Verification items for the finished model (mm, model axes). A direction names the side the tool comes from. Give positions to 0.01 mm unless a question says otherwise; leave off trailing zeros. Loops run counter-clockwise (first coordinate to the right, second up) from the corner with the lowest first, then second, coordinate; pieces in that order, holes last. Notation, with made-up numbers: (32, 50) - (79, 50) arc R23 ccw to (79, 71) - close; hole circle Ø9 at (-15.5, -2). An arc over 180 degrees is marked (long way). Use one line per item in the form item = value.
```python
from build123d import *

# Parameters (mm, degrees)
AUFSATZ_LINEAR_AUSTRAGEN1_DEPTH                      = 10
SCHNITT_LINEAR_AUSTRAGEN1_DEPTH                      = 8
SCHNITT_LINEAR_AUSTRAGEN2_DEPTH                      = 6
SKIZZE4_W                                            = 12
SKIZZE4_H                                            = 12
AUFSATZ_LINEAR_AUSTRAGEN2_DEPTH                      = 5
FASE1_SIZE                                           = 5
FORMSENKUNG_F_R_M4_LINSENSENKSCHRAUBE_MI_D           = 4.5
FORMSENKUNG_F_R_M4_LINSENSENKSCHRAUBE_MI_CSINK_D     = 9.4
FORMSENKUNG_F_R_M4_LINSENSENKSCHRAUBE_MI_CSINK_ANGLE = 90
VERRUNDUNG1_R                                        = 2
SKIZZE8_W                                            = 10.4
SKIZZE8_H                                            = 2
AUFSATZ_LINEAR_AUSTRAGEN3_DEPTH                      = 1
FASE2_SIZE                                           = 2


with BuildPart() as part:
    # Skizze1 → Aufsatz-Linear austragen1 (new body)
    with BuildSketch(Plane.XY):
        Polygon((-12, 0), (12, 0), (12, -12), (24, -12), (24, -24), (-24, -24), (-24, -12), (-12, -12), align=None)
    extrude(amount=AUFSATZ_LINEAR_AUSTRAGEN1_DEPTH)

    # Skizze2 → Schnitt-Linear austragen1 (cut)
    with BuildSketch(Plane.XY.offset(10)):
        Polygon((-5.2, -1), (-5.2, -7), (-24, -7), (-24, -24), (24, -24), (24, -7), (5.2, -7), (5.2, -1), align=None)
    extrude(amount=-SCHNITT_LINEAR_AUSTRAGEN1_DEPTH, mode=Mode.SUBTRACT)

    # Skizze3 → Schnitt-Linear austragen2 (cut)
    with BuildSketch(Plane(origin=(0, 0, 0), x_dir=(1, 0, 0), z_dir=(0, 1, 0))):
        with BuildLine():
            Line((-2.75, -2.8), (2.75, -2.8))
            ThreePointArc((2.75, -2.8), (4.5, -4.55), (2.75, -6.3))
            Line((2.75, -6.3), (-2.75, -6.3))
            ThreePointArc((-2.75, -6.3), (-4.5, -4.55), (-2.75, -2.8))
        make_face()
    extrude(amount=-SCHNITT_LINEAR_AUSTRAGEN2_DEPTH, mode=Mode.SUBTRACT)

    # Skizze4 → Aufsatz-Linear austragen2 (add)
    with BuildSketch(Plane.XY.offset(2)):
        with Locations((-18, -18)):
            Rectangle(SKIZZE4_W, SKIZZE4_H)
        with Locations((18, -18)):
            Rectangle(SKIZZE4_W, SKIZZE4_H)
    extrude(amount=AUFSATZ_LINEAR_AUSTRAGEN2_DEPTH)

    # Fase1
    fase1_edges = [part.edges().sort_by_distance(p)[0] for p in [
        (12, -18, 2),
        (-12, -18, 2),
    ]]
    chamfer(fase1_edges, length=FASE1_SIZE - 0.0001)  # a hair under: the kernel refuses the full size

    # Formsenkung für M4 Linsensenkschraube mit Schlitz1 (through all)
    with Locations(Plane.XY.offset(7)):
        with Locations((-18, -18), (18, -18)):
            CounterSinkHole(FORMSENKUNG_F_R_M4_LINSENSENKSCHRAUBE_MI_D / 2, FORMSENKUNG_F_R_M4_LINSENSENKSCHRAUBE_MI_CSINK_D / 2, counter_sink_angle=FORMSENKUNG_F_R_M4_LINSENSENKSCHRAUBE_MI_CSINK_ANGLE)

    # Verrundung1
    verrundung1_edges = [part.edges().sort_by_distance(p)[0] for p in [
        (24, -12, 3.5),
        (24, -24, 3.5),
        (-24, -24, 3.5),
        (-24, -12, 3.5),
    ]]
    fillet(verrundung1_edges, radius=VERRUNDUNG1_R)

    # Skizze8 → Aufsatz-Linear austragen3 (add)
    with BuildSketch(Plane.XY.offset(10)):
        with Locations((0, -2)):
            Rectangle(SKIZZE8_W, SKIZZE8_H)
    extrude(amount=-AUFSATZ_LINEAR_AUSTRAGEN3_DEPTH)

    # Fase2
    fase2_edges = [part.edges().sort_by_distance(p)[0] for p in [
        (0, -1, 9),
    ]]
    chamfer(fase2_edges, length=FASE2_SIZE - 0.0001)  # a hair under: the kernel refuses the full size


solid = part.part
```
1. Section check C-C, the plane z = 1.25. Record the cut outline in (x, y).
Result set:
outline = (-24, -22) arc R2 ccw to (-22, -24) - (22, -24) arc R2 ccw to (24, -22) - (24, -14) arc R2 ccw to (22, -12) - (12, -12) - (12, 0) - (-12, 0) - (-12, -12) - (-22, -12) arc R2 ccw to (-24, -14) - close; hole circle Ø4.5 at (-18, -18); hole circle Ø4.5 at (18, -18)
2. Scan lines: probe 1 along X at (y, z) = (-18, 0.95); probe 2 along Y at (x, z) = (18, 1.85); probe 3 along X at (y, z) = (-3.5, 9). Record each from-to range of solid material in increasing order.
Result set:
probe_1 = -24 to -20.25, -15.75 to 15.75, 20.25 to 24
probe_2 = -24 to -20.25, -15.75 to -12
probe_3 = -12 to -5.2, 5.2 to 12
3. Section check A-A, the plane x = 18. Record the cut outline in (y, z).
Result set:
outline = (-24, 0) - (-20.25, 0) - (-20.25, 4.55) - (-22.7, 7) - (-24, 7) - close; (-15.75, 0) - (-12, 0) - (-12, 7) - (-13.3, 7) - (-15.75, 4.55) - close
4. Depth check by flat-ended pin: pin 1 Ø1 at (y, z) = (-10.5, 4) entering from -X; pin 2 Ø3.5 at (x, z) = (14, 4.5) entering from +Y; pin 3 Ø2 at (y, z) = (-6, 1) entering from -X; pin 4 Ø3.5 at (x, y) = (-16, -19.5) entering from +Z. Enter the tip coordinate at first touch or a pass-through.
Result set:
pin_1 = through
pin_2 = -12
pin_3 = -12
pin_4 = 6.55
5. Draft check along X on faces 1 (the cylindrical face through (-23.4, -23.43, 3.55)), 2 (the flat face through (0, -14, 0)), 3 (the cylindrical face through (-4.5, -0.5, 4.6)). Enter one of: released by +X, released by -X, zero draft, split by the parting line, or undercut.
Result set:
face_1 = released by -X
face_2 = zero draft
face_3 = undercut
6. Section check B-B, the plane z = 3.75. Record the cut outline in (x, y).
Result set:
outline = (-24, -22) arc R2 ccw to (-22, -24) - (-8.75, -24) - (-8.75, -12) - (-22, -12) arc R2 ccw to (-24, -14) - close; (-12, -7) - (-5.2, -7) - (-5.2, -1) - (-4.31, -1) - (-4.31, 0) - (-12, 0) - close; (4.31, -1) - (5.2, -1) - (5.2, -7) - (12, -7) - (12, 0) - (4.31, 0) - close; (8.75, -24) - (22, -24) arc R2 ccw to (24, -22) - (24, -14) arc R2 ccw to (22, -12) - (8.75, -12) - close; hole circle Ø4.5 at (-18, -18); hole circle Ø4.5 at (18, -18)
7. Tool access check on faces 4 (the flat face through (-10, -18, 5)), 5 (the flat face through (0, -0.5, 2.8)), 6 (the flat face through (-16, -12, 3)). Record the directions out of +Z, -Z, +X, -X, +Y, -Y that give a thin tool (end or side, any length) a straight path to the whole face; none if there is none.
Result set:
face_4 = +Z, -Y
face_5 = +Y, -Y
face_6 = +Z, -X
8. Section check D-D, the plane y = -3.5. Record the cut outline in (x, z).
Result set:
outline = (-12, 0) - (12, 0) - (12, 10) - (5.2, 10) - (5.2, 2) - (-5.2, 2) - (-5.2, 10) - (-12, 10) - close
